The figure shows three views and two pictorial views of one solid part (mm, origin at its lowest corner). Answer the questions. A direction names the side the tool comes from. Round coordinates to 2 decimals unless told otherwise and drop trailing zeros. Order: outer loops, then holes, each group sorted by start corner. A loop starts at its lowest first (then second) coordinate and runs counter-clockwise, first axis right, second up. Notation, with made-up numbers: (84.5, 64.5) -> (137.5, 64.5) arc R20 cw to (137.5, 81.5) -> close; hole circle Ø10 at (7.5, 31). An arc over 180 degrees is marked (long way). One line per item, written item: value. Start each with the question number.
1. Section D-D (z = 9) is taken. Give the vertices of the cut face in (x, y), then the cut area to 3 significant figures.
2. The mould has two halves that part along Z. Classify the marked faces 3, 4, 5 and 6: released by +Z, released by -Z, zero draft, split by the parting line, or undercut.
3. Section B-B (y = 8.1) is taken. Give the vertices of the cut face in (x, z), then the cut area to 3 significant figures.
4. For the marked faces 1 and 2, determine the directions among +Z, -Z, +X, -X, +Y, -Y from which every point of the face is accessible in a straight line to the end or side of a thin tool.
5. Section A-A (z = 4) is taken. Give the vertices of the cut face in (x, y).
6. Consider line 1 (Z direction, x = 1.2, y = 8.1); line 2 (X direction, y = 7, z = 6.5); line 3 (X direction, y = 10.5, z = 10.75). Determine where each line is inside the solid, lowest interval first.
7. Section C-C (y = 11.5) is taken. Give the vertices of the cut face in (x, z).
8. Flat-ended cylindrical pins translate along their axes: pin 1 Ø3 at (y, z) = (3.5, 2) entering from -X; pin 2 Ø2.5 at (y, z) = (10, 2) entering from +X; pin 3 Ø4 at (x, y) = (6.5, 11) entering from +Z; pin 4 Ø2 at (x, z) = (12.5, 10.5) entering from -Y. Find the tip coordinate at first contact, or state that the pin passes through.
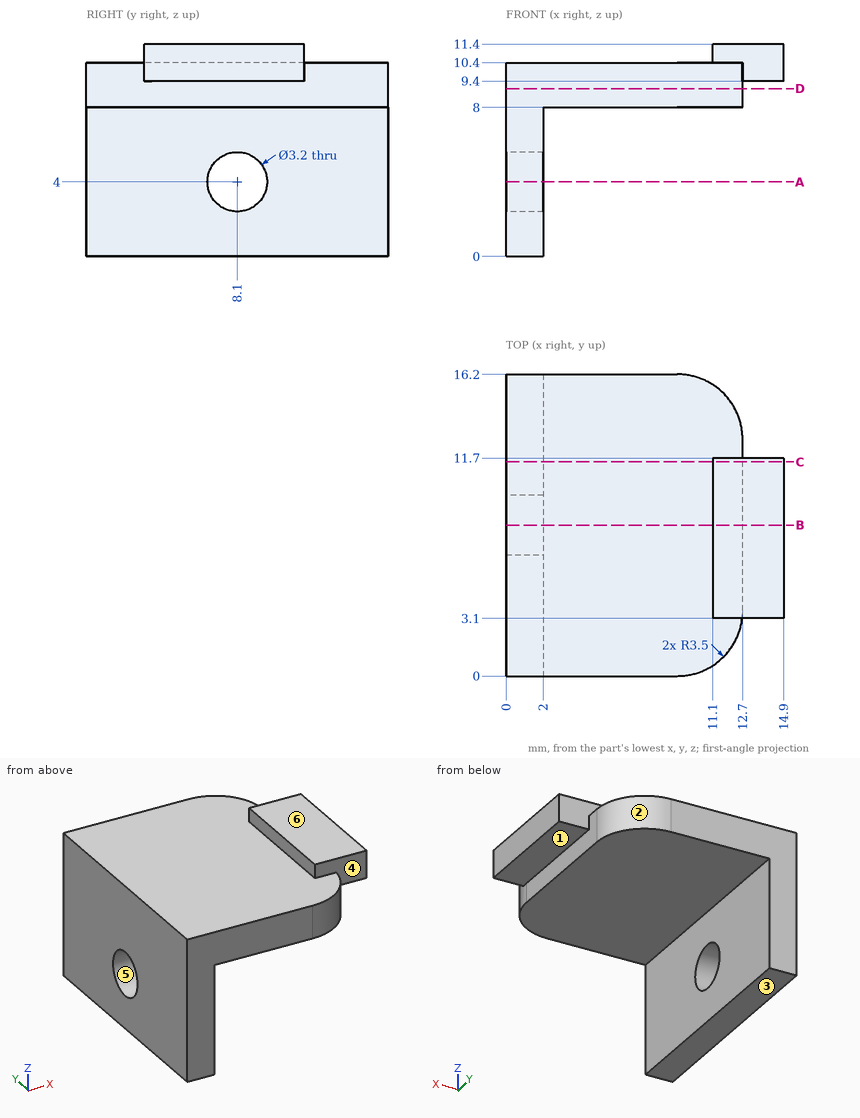
Answer:
1. outline: (0, 0) -> (9.2, 0) arc R3.5 ccw to (12.7, 3.5) -> (12.7, 12.7) arc R3.5 ccw to (9.2, 16.2) -> (0, 16.2) -> close
1. area: 200 mm^2
2. face 3: released by -Z
2. face 4: zero draft
2. face 5: undercut
2. face 6: released by +Z
3. outline: (0, 0) -> (2, 0) -> (2, 2.4) -> (0, 2.4) -> close; (0, 5.6) -> (2, 5.6) -> (2, 8) -> (12.7, 8) -> (12.7, 9.4) -> (14.9, 9.4) -> (14.9, 11.4) -> (11.1, 11.4) -> (11.1, 10.4) -> (0, 10.4) -> close
3. area: 46.1 mm^2
4. face 1: -Z, +X, +Y, -Y
4. face 2: +Z, -Z, +X, +Y
5. outline: (0, 0) -> (2, 0) -> (2, 6.5) -> (0, 6.5) -> close; (0, 9.7) -> (2, 9.7) -> (2, 16.2) -> (0, 16.2) -> close
6. line 1: 0 to 2.4, 5.6 to 10.4
6. line 2: 0 to 2
6. line 3: 11.1 to 14.9
7. outline: (0, 0) -> (2, 0) -> (2, 8) -> (12.7, 8) -> (12.7, 9.4) -> (14.9, 9.4) -> (14.9, 11.4) -> (11.1, 11.4) -> (11.1, 10.4) -> (0, 10.4) -> close
8. pin 1: x = 0
8. pin 2: x = 2
8. pin 3: z = 10.4
8. pin 4: y = 0.87
